from build123d import *

# Parameters (mm, degrees)
SKETCH_1_R               = 6.5
SKETCH_1_R_2             = 5.375
EXTRUDE_1_DEPTH          = 13
SKETCH_2_W               = 1.65
SKETCH_2_H               = 11.5
CUT_EXTRUDE_1_DEPTH      = 6.5
PATTERN_CIRCULAR_1_COUNT = 14


with BuildPart() as part:
    # Эскиз1 → Бобышка-Вытянуть1 (new body)
    with BuildSketch(Plane.XY):
        with Locations(Location((0, 0, 0), (0, 0, 180))):
            Circle(SKETCH_1_R)
        with Locations(Location((0, 0, 0), (0, 0, 180))):
            Circle(SKETCH_1_R_2, mode=Mode.SUBTRACT)
    extrude(amount=EXTRUDE_1_DEPTH)

    # Эскиз2 → Вырез-Вытянуть1 (cut)
    with BuildSketch(Plane(origin=(0, 0, 0), x_dir=(1, 0, 0), z_dir=(0, 1, 0))):
        with Locations((0, -6.5)):
            Rectangle(SKETCH_2_W, SKETCH_2_H)
    cut_extrude_1 = extrude(amount=-CUT_EXTRUDE_1_DEPTH, mode=Mode.SUBTRACT)

    # Круговой массив1: Вырез-Вытянуть1 ×14 about axis
    pattern_circular_1_axis = Axis((0, 0, 0), (0, 0, 1))
    for i in range(1, PATTERN_CIRCULAR_1_COUNT):
        add(cut_extrude_1.rotate(pattern_circular_1_axis, i * 360 / PATTERN_CIRCULAR_1_COUNT), mode=Mode.SUBTRACT)


solid = part.part
CAD build for the part. Positions are in the model's coordinates, mm. A direction names the side the tool comes from. Coordinates: 2 decimals unless noted, no trailing zeros. Order: outer loops, then holes, each group sorted by start corner. A loop starts at its lowest first (then second) coordinate and runs counter-clockwise, first axis right, second up.
Item 1: Band-saw the part on A-A on x = 0. List the corners of the cut face in (y, z) (3 decimals).
Check sheet entries:
outline: (-6.5, 0) - (-5.375, 0) - (-5.375, 0.75) - (-6.5, 0.75) - close; (-6.5, 12.25) - (-5.375, 12.25) - (-5.375, 13) - (-6.5, 13) - close; (5.375, 0) - (6.5, 0) - (6.5, 0.75) - (5.375, 0.75) - close; (5.375, 12.25) - (6.5, 12.25) - (6.5, 13) - (5.375, 13) - close
Item 2: Band-saw the part on B-B on y = 0. List the corners of the cut face in (x, z) (3 decimals), plus the area to 4 significant figures.
Check sheet entries:
outline: (-6.5, 0) - (-5.375, 0) - (-5.375, 13) - (-6.5, 13) - close; (5.375, 0) - (6.5, 0) - (6.5, 13) - (5.375, 13) - close
area: 29.25 mm2
Item 3: Drill centre lines: L1, parallel to Z at x = 5.5, y = -2; L2, parallel to Y at x = 5.5, z = 1; L3, parallel to Y at x = 4, z = 12. Where is each one in solid material? Low to high.
Check sheet entries:
L1: z = 0 to 0.75, 12.25 to 13
L2: y = -3.33 to -2.1, -0.41 to 0.41, 2.1 to 3.33
L3: y = -5.12 to -4.25, 4.25 to 5.12
Item 4: Pin check, flat tips, straight feed: pin 1 Ø2 at (y, z) = (4, 8) entering from -X; pin 2 Ø0.6 at (y, z) = (-6, 8) entering from -X; pin 3 Ø1.5 at (x, z) = (3, 7) entering from -Y. Stop position of each tip, or through.
Check sheet entries:
pin 1: stops at x = -5.77
pin 2: stops at x = -2.05
pin 3: stops at y = -5.45
Item 5: 3-axis set-ups, long thin cutter, end or side, ignore diameter. For faces 1 (the face through (0, -6, 0.75)), 2 (the face through (-3.29, 4.93, 6.58)), 3 (the face through (-3, -5, 0.75)), 4 (the face through (4.08, 4.31, 6.58)): which of +Z, -Z, +X, -X, +Y, -Y reach the whole face in a straight line?
Check sheet entries:
face 1: +Y, -Y
face 2: +Y
face 3: none
face 4: +X
Item 6: Band-saw the part on D-D on z = 2. Give the number of separate pieces and of enclosed holes in the cut face, plus the area to 3 significant figures.
Check sheet entries:
separate pieces: 14
enclosed holes: 0
area: 15.9 mm2
Item 7: Band-saw the part on C-C on x = -4. List the corners of the cut face in (y, z).
Check sheet entries:
outline: (-5.12, 0) - (-3.59, 0) - (-3.59, 0.75) - (-4.25, 0.75) - (-4.25, 12.25) - (-3.59, 12.25) - (-3.59, 13) - (-5.12, 13) - close; (3.59, 0) - (5.12, 0) - (5.12, 13) - (3.59, 13) - (3.59, 12.25) - (4.25, 12.25) - (4.25, 0.75) - (3.59, 0.75) - close
